```python
from build123d import *

# Parameters (mm, degrees)
F0_R     = 2.1
F1_DEPTH = 3


with BuildPart() as f1:
    # F0 (on Top) → F1 (new body)
    with BuildSketch(Plane.XY):
        with BuildLine():
            Line((-41, 14.5), (-41, -5.5))
            ThreePointArc((-41, -5.5), (-28.5, -18), (-16, -5.5))
            Line((-16, -5.5), (-16, 0))
            ThreePointArc((-16, 0), (0, 16), (16, 0))
            Line((16, 0), (16, -5.5))
            ThreePointArc((16, -5.5), (28.5, -18), (41, -5.5))
            Line((41, -5.5), (41, 14.5))
            ThreePointArc((41, 14.5), (31.825248, 33.967169), (17.5, 50.027492))
            ThreePointArc((17.5, 50.027492), (0, 53), (-17.5, 50.027492))
            ThreePointArc((-17.5, 50.027492), (-31.825248, 33.967169), (-41, 14.5))
        make_face()
        with Locations((-28.5, 0)):
            Circle(F0_R, mode=Mode.SUBTRACT)
        with Locations((28.5, 0)):
            Circle(F0_R, mode=Mode.SUBTRACT)
    extrude(amount=F1_DEPTH)


solid = f1.part
```
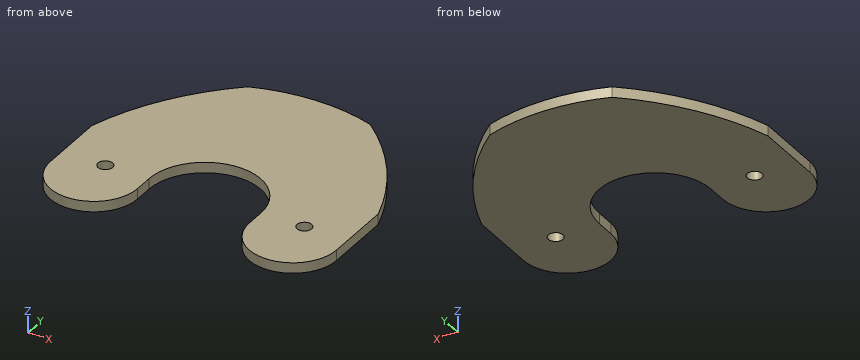
The model under review builds one solid part; all positions refer to its coordinate system, in mm. Round coordinates to 2 decimals unless told otherwise and drop trailing zeros. Order: outer loops, then holes, each group sorted by start corner. A loop starts at its lowest first (then second) coordinate and runs counter-clockwise, first axis right, second up. Notation, with made-up numbers: (36, 62) -> (69, 62) arc R17 ccw to (69, 77) -> close; hole circle Ø8 at (53.25, 89). An arc over 180 degrees is marked (long way). Use a Markdown table: item, result.
Q1. For line 1 (Y direction, x = -28, z = 2.5); line 2 (Y direction, x = -28.5, z = 1.8); line 3 (X direction, y = 31, z = 0.75), list the stretches that pass through material, from the lowest coordinate up.
Values:
| item | result |
|---|---|
| line 1 | y = -17.99 to -2.04, 2.04 to 39.24 |
| line 2 | y = -18 to -2.1, 2.1 to 38.6 |
| line 3 | x = -33.69 to 33.69 |
Q2. We need section C-C on x = 28.5. Write out the cut boundary in (y, z).
Values:
| item | result |
|---|---|
| outline | (-18, 0) -> (-2.1, 0) -> (-2.1, 3) -> (-18, 3) -> close; (2.1, 0) -> (38.6, 0) -> (38.6, 3) -> (2.1, 3) -> close |
Q3. We need section A-A on z = 1. Write out the cut boundary in (x, y).
Values:
| item | result |
|---|---|
| outline | (-41, -5.5) arc R12.5 ccw to (-16, -5.5) -> (-16, 0) arc R16 cw to (16, 0) -> (16, -5.5) arc R12.5 ccw to (41, -5.5) -> (41, 14.5) arc R75 ccw to (17.5, 50.03) arc R53 ccw to (-17.5, 50.03) arc R75 ccw to (-41, 14.5) -> close; hole circle Ø4.2 at (-28.5, 0); hole circle Ø4.2 at (28.5, 0) |
Q4. Clearance check with a flat-ended pin moving along its axis: P1, Ø12, axis at x = -22.5, y = 30, coming from the -Z side. State where the tip first meets the part, or that it passes through.
Values:
| item | result |
|---|---|
| P1 | stops at z = 0 |
Q5. We need section B-B on y = 9. Write out the cut boundary in (x, z).
Values:
| item | result |
|---|---|
| outline | (-41, 0) -> (-13.23, 0) -> (-13.23, 3) -> (-41, 3) -> close; (13.23, 0) -> (41, 0) -> (41, 3) -> (13.23, 3) -> close |
Q6. We need section D-D on x = 0. Write out the cut boundary in (y, z).
Values:
| item | result |
|---|---|
| outline | (16, 0) -> (53, 0) -> (53, 3) -> (16, 3) -> close |
